For this review, take the finished solid that the model builds, in its own axes (mm). A direction names the side the tool comes from. Round coordinates to 2 decimals unless told otherwise and drop trailing zeros. Loops run counter-clockwise (first coordinate to the right, second up) from the corner with the lowest first, then second, coordinate; pieces in that order, holes last.
1) Take a section at D-D (x = 12). State the section outline as (y, z) points, then the cut area to 3 significant figures.
2) Wall thickness on L1, parallel to Y at x = 11.5, z = 0; L2, parallel to Y at x = -17, z = 14; L3, parallel to X at y = 17, z = -15.5: over which ranges is each line inside the solid? List them lowest first.
3) Mouldability with a two-part tool opening along Z and no side actions: class faces 1 (the flat face through (0, 20.701, 0)), 2 (the cylindrical face through (13.39, 30.67, -0.06)), 3 (the cylindrical face through (15.048, 32.897, -3.098)) as pulls with the +Z half, pulls with the -Z half, needs draft (parallel to the pull), parting line crosses it, or undercut.
4) Take a section at A-A (z = 0). State the section outline as (x, y) points, then the cut area to 3 significant figures.
5) Take a section at B-B (x = 0). State the section outline as (y, z) points, then the cut area to 3 significant figures.
6) Insertion check: pin 1 (12 mm diameter, centred on x = 3.5, y = 34.5, fed in from +Z); pin 2 (4 mm diameter, centred on x = 15.5, y = 23.5, fed in from -Z); pin 3 (4 mm diameter, centred on x = 16, y = 4.5, fed in from -Z); pin 4 (4 mm diameter, centred on y = 12, z = 12.5, fed in from +X). Each pin has a flat end and moves straight along its axis. Give the tip position at first contact, or say it passes through.
7) Take a section at C-C (y = 18). State the section outline as (x, z) points, then the cut area to 3 significant figures.
8) Tool access review of faces 4 (the cylindrical face through (18.44, 22.87, 1.58)), 5 (the flat face through (0, 0, 0)): name each direction out of +Z, -Z, +X, -X, +Y, -Y from which nothing blocks a thin tool from reaching the whole face with its end or side.
Autodesk Inventor part; units mm, degrees
ref_plane "YZ Plane" through (0, 0, 0) normal (1, 0, 0) x (0, 1, 0)
ref_plane "XZ Plane" through (0, 0, 0) normal (0, 1, 0) x (-1, 0, 0)
ref_plane "XY Plane" through (0, 0, 0) normal (0, 0, 1) x (1, 0, 0)
sketch "Sketch1" plane through (0, 0, 0) normal (0, 1, 0) x (-1, 0, 0)
  circle A0 centre (0, 0) radius 24.638
  dimension "d0" = 49.276
extrude "Extrusion1" add sketch "Sketch1" along normal blind 20.701
sketch "Sketch2" plane through (0, 20.701, 0) normal (0, 1, 0) x (1, 0, 0)
  circle A0 centre (13.4366, 0) radius 3.4925
  point P0 (0, 0)
  dimension "d3" = 6.985
  dimension "d4" = 13.4366
extrude "Extrusion2" add sketch "Sketch2" along normal blind 20.2184
sketch "Sketch3" plane through (0, 20.701, 0) normal (0, 1, 0) x (1, 0, 0)
  circle A0 centre (13.4366, 0) radius 3.4925
  circle A1 centre (13.4366, 0) radius 5.2451
  point P0 (0, 0)
  dimension "d7" = 10.4902
extrude "Extrusion3" add sketch "Sketch3" along normal blind 4.3942 contours A0 | A1
sketch "Sketch4" plane through (0, 0, 0) normal (1, 0, 0) x (0, 1, 0)
  circle A0 centre (32.131, 0) radius 1.4605
  line L0 (20.701, -24.638) -> (20.701, 24.638)
  point P0 (0, 0)
  dimension "d10" = 2.921
  dimension "d11" = 11.43
extrude "Extrusion4" cut sketch "Sketch4" along normal through all
properties part number "24W_motor"
Response:
1. outline: (0, -21.52) - (20.7, -21.52) - (20.7, -5.04) - (25.1, -5.04) - (25.1, -3.18) - (40.92, -3.18) - (40.92, 3.18) - (25.1, 3.18) - (25.1, 5.04) - (20.7, 5.04) - (20.7, 21.52) - (0, 21.52) - close; hole circle Ø2.92 at (32.13, 0)
1. area: 1,030 mm2
2. L1: y = 0 to 30.67, 33.59 to 40.92
2. L2: y = 0 to 20.7
2. L3: x = -19.15 to 19.15
3. face 1: needs draft
3. face 2: undercut
3. face 3: parting line crosses it
4. outline: (-24.64, 0) - (24.64, 0) - (24.64, 20.7) - (18.68, 20.7) - (18.68, 25.1) - (16.93, 25.1) - (16.93, 30.67) - (9.94, 30.67) - (9.94, 25.1) - (8.19, 25.1) - (8.19, 20.7) - (-24.64, 20.7) - close; (9.94, 33.59) - (16.93, 33.59) - (16.93, 40.92) - (9.94, 40.92) - close
4. area: 1,160 mm2
5. outline: (0, -24.64) - (20.7, -24.64) - (20.7, 24.64) - (0, 24.64) - close
5. area: 1,020 mm2
6. pin 1: passes through
6. pin 2: stops at z = -5.24
6. pin 3: stops at z = -20.27
6. pin 4: stops at x = 22.29
7. outline: circle Ø49.28 at (0, 0)
7. area: 1,910 mm2
8. face 4: +Y
8. face 5: +Z, -Z, +X, -X, -Y
